Verification items for this drawing (mm, ordinates from the low corner). Round coordinates to 2 decimals unless told otherwise and drop trailing zeros. Loops run counter-clockwise (first coordinate to the right, second up) from the corner with the lowest first, then second, coordinate; pieces in that order, holes last. Notation, with made-up numbers: M 12.25,8.25 L 71.25,8.25 A25 cw 71.25,20.25 Z; hole C 19,-1 d6. An arc over 180 degrees is marked long. Write item = value, one per line. Start each with the question number.
(1) Scan lines: L1, parallel to X at y = 60, z = 5.5; L2, parallel to Y at x = 73.5, z = 21.5. Record each from-to range of solid material in increasing order. Write a range as from..to.
(2) Cross-section at A-A on z = 10.5. Record the boundary of the cut face in (x, y).
(3) Cross-section at D-D on y = 20. Record the boundary of the cut face in (x, z).
(4) Cross-section at B-B on y = 40. Record the boundary of the cut face in (x, z).
(5) Cross-section at C-C on x = 60. Record the boundary of the cut face in (y, z), plus the area to 3 significant figures.
(6) Go/stop test with flat-tipped pins: P1, Ø4.5, axis at x = 26.5, z = 14, coming from the -Y side; P2, Ø9, axis at x = 60, y = 60, coming from the -Z side. Record where each tip stops, or that it passes through.
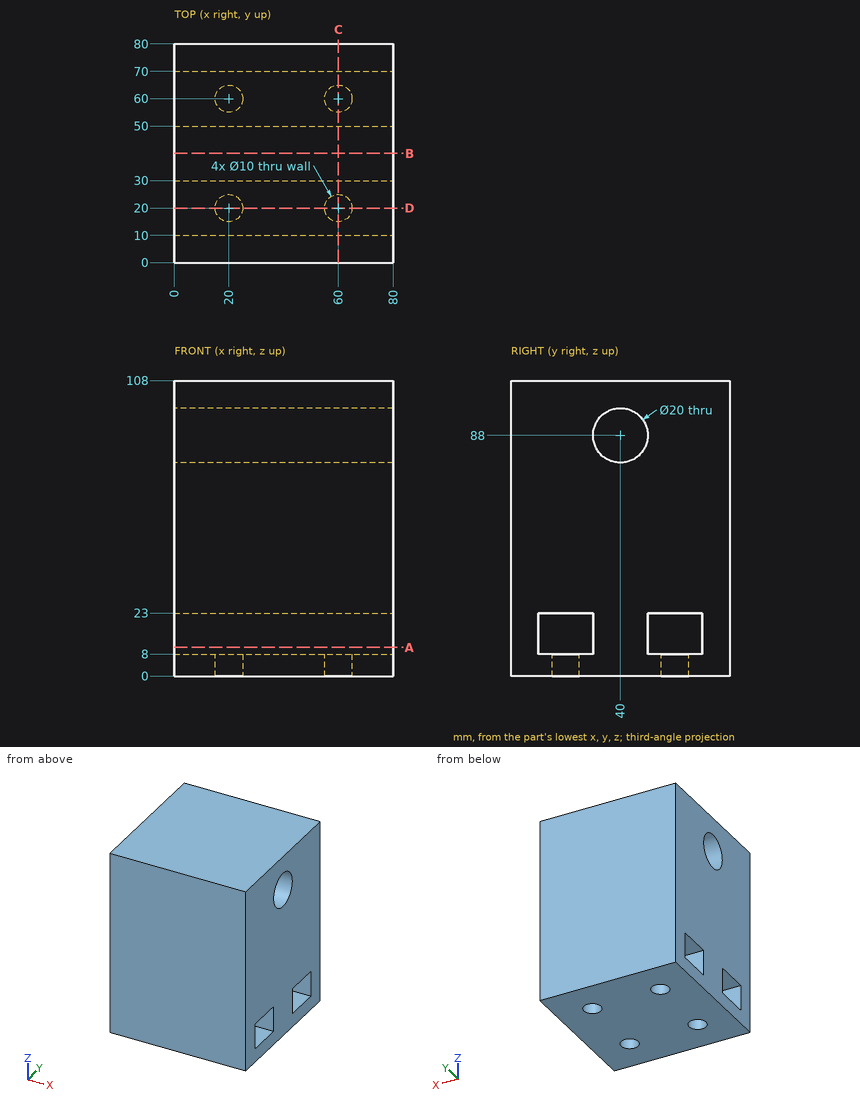
Result:
q1.L1 = 0..15, 25..55, 65..80
q1.L2 = 0..10, 30..50, 70..80
q2.outline = M 0,0 L 80,0 L 80,10 L 0,10 Z; M 0,30 L 80,30 L 80,50 L 0,50 Z; M 0,70 L 80,70 L 80,80 L 0,80 Z
q3.outline = M 0,0 L 15,0 L 15,8 L 0,8 Z; M 0,23 L 80,23 L 80,108 L 0,108 Z; M 25,0 L 55,0 L 55,8 L 25,8 Z; M 65,0 L 80,0 L 80,8 L 65,8 Z
q4.outline = M 0,0 L 80,0 L 80,78 L 0,78 Z; M 0,98 L 80,98 L 80,108 L 0,108 Z
q5.outline = M 0,0 L 15,0 L 15,8 L 10,8 L 10,23 L 30,23 L 30,8 L 25,8 L 25,0 L 55,0 L 55,8 L 50,8 L 50,23 L 70,23 L 70,8 L 65,8 L 65,0 L 80,0 L 80,108 L 0,108 Z; hole C 40,88 d20
q5.area = 7,570 mm^2
q6.P1 = 0
q6.P2 = 23
